```python
from build123d import *

# Parameters (mm, degrees)
SKETCH1_R           = 38
SKETCH1_R_2         = 1
BOSS_EXTRUDE1_DEPTH = 1


with BuildPart() as part:
    # Sketch1 → Boss-Extrude1 (new body)
    with BuildSketch(Plane(origin=(0, 0, 0), x_dir=(1, 0, 0), z_dir=(0, 1, 0))):
        with Locations(Location((0, 0, 0), (0, 0, 270))):
            Circle(SKETCH1_R)
        with Locations(Location((28.5, 0, 0), (0, 0, 270))):
            Circle(SKETCH1_R_2, mode=Mode.SUBTRACT)
        with Locations(Location((-28.5, 0, 0), (0, 0, 270))):
            Circle(SKETCH1_R_2, mode=Mode.SUBTRACT)
        with Locations(Location((13.5, 13.5, 0), (0, 0, 270))):
            Circle(SKETCH1_R_2, mode=Mode.SUBTRACT)
        with Locations(Location((13.5, -13.5, 0), (0, 0, 270))):
            Circle(SKETCH1_R_2, mode=Mode.SUBTRACT)
        with Locations(Location((-9.5, 0, 0), (0, 0, 270))):
            Circle(SKETCH1_R_2, mode=Mode.SUBTRACT)
    extrude(amount=-BOSS_EXTRUDE1_DEPTH)


solid = part.part
```
Part model, mm, in its own coordinate system. Coordinates: 2 decimals unless noted, no trailing zeros. Loops run counter-clockwise (first coordinate to the right, second up) from the corner with the lowest first, then second, coordinate; pieces in that order, holes last. Notation, with made-up numbers: (-16, 3.5) - (12, 3.5) arc R30 cw to (12, 29.5) - close; hole circle Ø3 at (25.5, -20.5). An arc over 180 degrees is marked (long way). Write item = value, one per line. Start each with the question number.
Item 1: Wall check: L1, parallel to X at y = -0.5, z = 0; L2, parallel to Z at x = 1, y = -0.1; L3, parallel to X at y = -0.35, z = -13.5. Give the ranges that are in metal, low to high. Write a range as from..to.
Item 2: Cut at C-C, the plane z = -13.5. Give the cut face in (x, y), and give its area (3 significant figures).
Item 3: Mould opens along X. For faces 1 (the cylindrical face through (-8.51, -0.49, -0.13)), 2 (the cylindrical face through (-23.122, -0.493, -30.156)), 3 (the cylindrical face through (12.61, -0.49, 13.96)), 4 (the flat face through (1, -1, -1)) say: released by +X, released by -X, zero draft, split by the parting line, or undercut.
Item 4: Flat gauge pin, fed straight in: pin 1 Ø1.8 at (x, z) = (-9.5, 0) entering from +Y. Where does the tip first touch, or does it go through?
Item 5: Cut at B-B, the plane y = -0.3. Give the cut face in (x, z), and give its area (3 significant figures).
Item 6: Cut at D-D, the plane x = -17. Give the cut face in (y, z), and give its area (3 significant figures).
Item 7: Cut at A-A, the plane x = -28.5. Give the cut face in (y, z), and give its area (3 significant figures).
The answers:
q1.L1 = -38..-29.5, -27.5..-10.5, -8.5..27.5, 29.5..38
q1.L2 = -37.99..37.99
q1.L3 = -35.52..12.5, 14.5..35.52
q2.outline = (-35.52, -1) - (12.5, -1) - (12.5, 0) - (-35.52, 0) - close; (14.5, -1) - (35.52, -1) - (35.52, 0) - (14.5, 0) - close
q2.area = 69.0 mm2
q3.face_1 = undercut
q3.face_2 = split by the parting line
q3.face_3 = undercut
q3.face_4 = zero draft
q4.pin_1 = through
q5.outline = circle Ø76 at (0, 0); hole circle Ø2 at (-28.5, 0); hole circle Ø2 at (-9.5, 0); hole circle Ø2 at (13.5, -13.5); hole circle Ø2 at (13.5, 13.5); hole circle Ø2 at (28.5, 0)
q5.area = 4,520 mm2
q6.outline = (-1, -33.99) - (0, -33.99) - (0, 33.99) - (-1, 33.99) - close
q6.area = 68.0 mm2
q7.outline = (-1, -25.13) - (0, -25.13) - (0, -1) - (-1, -1) - close; (-1, 1) - (0, 1) - (0, 25.13) - (-1, 25.13) - close
q7.area = 48.3 mm2
